Design review of the part built by this model. Coordinates are the model's own, in mm. Face numbers are marked on the shaded views. A direction names the side the tool comes from. Coordinates: 2 decimals unless noted, no trailing zeros. Loops run counter-clockwise (first coordinate to the right, second up) from the corner with the lowest first, then second, coordinate; pieces in that order, holes last. Notation, with made-up numbers: (-25, 76.25) - (-7, 76.25) arc R24 cw to (-7, 100.25) - close; hole circle Ø1 at (-26, 51.5). An arc over 180 degrees is marked (long way). Return JSON: item names as keys, results as strings. Group by question number.
from build123d import *

# Parameters (mm, degrees)
F0_W     = 60
F0_H     = 30
F1_DEPTH = 40
F2_W     = 28.0448670685
F2_H     = 40
F3_DEPTH = 25.4
F3_TAPER = 15
F4_R     = 3.2869844705
F5_DEPTH = 25


# Not quite as in the source:
# - a feature names something its author has since deleted; it is built from what else it names


with BuildPart() as f1:
    # F0 (on Front) → F1 (new body)
    with BuildSketch(Plane.XZ):
        with Locations((-1.9551329315, 8.1626253676)):
            Rectangle(F0_W, F0_H)
    extrude(amount=F1_DEPTH)

    # F2 (on face) → F3 (join)
    with BuildSketch(Plane.XY.offset(23.1626253676)):
        with Locations((14.0224335343, -20)):
            Rectangle(F2_W, F2_H)
    extrude(amount=F3_DEPTH, taper=F3_TAPER)

    # F4 (on face) → F5 (cut)
    with BuildSketch(Plane.XY.offset(48.5626253676)):
        with Locations((14.0224335343, -20)):
            Circle(F4_R)
    extrude(amount=-F5_DEPTH, mode=Mode.SUBTRACT)


solid = f1.part
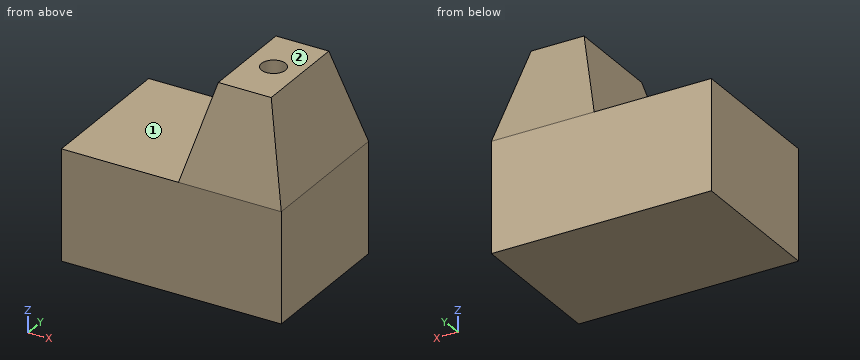
Item 1: Add section A-A (y = -12). State the section outline as (x, z) points.
Item 2: To check wall thickness, follow line 1 (Z direction, x = -4, y = -14.5); line 2 (X direction, y = -31, z = 38); line 3 (X direction, y = -4.5, z = 39). State the ranges of each line that lie inside material, in increasing order. Write a range as from..to.
Item 3: Add section D-D (y = -20). State the section outline as (x, z) points.
Item 4: For P1, Ø2, axis at x = 14.5, y = -19, coming from the +Z side; P2, Ø8, axis at y = -8.5, z = 26, coming from the -X side; P3, Ø16, axis at x = -24, y = -24.5, coming from the +Z side, all flat-tipped, find the tip position at first contact; note any pin that passes through.
Item 5: For the marked faces 1 and 2, list the 3-axis set-ups (+Z, -Z, +X, -X, +Y, -Y) from which the entire face can be reached by the end or side of a thin tool; tool diameter is ignored.
Item 6: Add section C-C (z = 32). State the section outline as (x, y) points, then the cut area to 3 significant figures.
Item 7: Add section B-B (x = 13). State the section outline as (y, z) points.
Answers below:
{
 "1": {"outline": "(-31.96, -6.84) - (28.04, -6.84) - (28.04, 23.16) - (21.24, 48.56) - (6.81, 48.56) - (0, 23.16) - (-31.96, 23.16) - close"},
 "2": {"line 1": "z = -6.84..23.16", "line 2": "x = 3.98..24.07", "line 3": "x = 4.24..23.8"},
 "3": {"outline": "(-31.96, -6.84) - (28.04, -6.84) - (28.04, 23.16) - (21.24, 48.56) - (17.31, 48.56) - (17.31, 23.56) - (10.74, 23.56) - (10.74, 48.56) - (6.81, 48.56) - (0, 23.16) - (-31.96, 23.16) - close"},
 "4": {"P1": "stops at z = 23.56", "P2": "stops at x = -31.96", "P3": "stops at z = 23.16"},
 "5": {"face 1": "+Z, -X, +Y, -Y", "face 2": "+Z, +X, -X, +Y, -Y"},
 "6": {"outline": "(2.37, -37.63) - (25.68, -37.63) - (25.68, -2.37) - (2.37, -2.37) - close; hole circle Ø6.57 at (14.02, -20)", "area": "788 mm^2"},
 "7": {"outline": "(-40, -6.84) - (0, -6.84) - (0, 23.16) - (-6.81, 48.56) - (-16.88, 48.56) - (-16.88, 23.56) - (-23.12, 23.56) - (-23.12, 48.56) - (-33.19, 48.56) - (-40, 23.16) - close"}
}
